```python
from build123d import *

# Parameters (mm, degrees)
F0_W     = 25.4
F0_H     = 25.4
F1_DEPTH = 25.4
F3_DEPTH = 23.368
F2_W     = 2.54
F2_H     = 15.24
F4_DEPTH = 20.32


with BuildPart() as f1:
    # F0 (on Top) → F1 (new body)
    with BuildSketch(Plane.XY):
        Rectangle(F0_W, F0_H)
    extrude(amount=F1_DEPTH)

    # F2 (on face) → F3 (cut)
    with BuildSketch(Plane(origin=(0, 0, 0), x_dir=(1, 0, 0), z_dir=(0, 0, -1))):
        Polygon((10.16, -7.62), (10.16, 7.62), (10.16, 10.668), (7.62, 10.668), (7.62, -10.668), (10.16, -10.668), align=None)
    extrude(amount=-F3_DEPTH, mode=Mode.SUBTRACT)

    # F2 (on face) → F4 (cut)
    with BuildSketch(Plane(origin=(0, 0, 0), x_dir=(1, 0, 0), z_dir=(0, 0, -1))):
        with Locations((11.43, 0)):
            Rectangle(F2_W, F2_H)
    extrude(amount=-F4_DEPTH, mode=Mode.SUBTRACT)


solid = f1.part
```
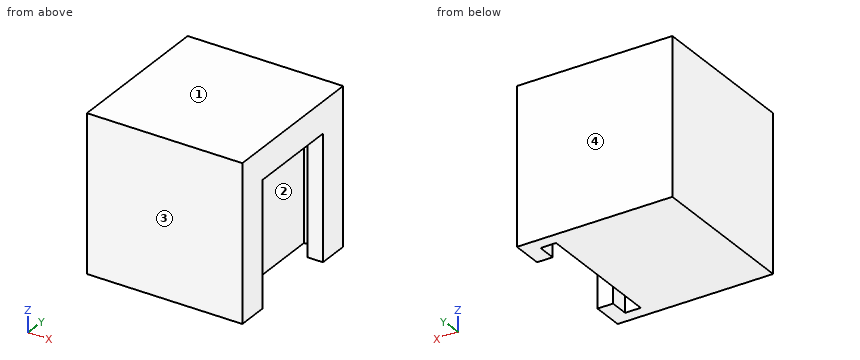
Check sheet for the modelled part. Datum: model origin and axes. Units: mm. Face numbers are marked on the shaded views. Coordinates: 2 decimals unless noted, no trailing zeros. Write each loop counter-clockwise with the first axis right and the second up, starting at its lowest first coordinate (ties: lowest second). Pieces come first, ordered by that corner, then holes. Notation, with made-up numbers: (11, 69.25) -> (55, 69.25) arc R32 ccw to (55, 97.25) -> close; hole circle Ø9 at (37, -3). An arc over 180 degrees is marked (long way). Use a Markdown table: item, result.
1. Sectioned sample at C-C (y = 9.5). Enter the section's corners in (x, z), plus the area to 3 significant figures.
Reported:
| item | result |
|---|---|
| outline | (-12.7, 0) -> (7.62, 0) -> (7.62, 23.37) -> (10.16, 23.37) -> (10.16, 0) -> (12.7, 0) -> (12.7, 25.4) -> (-12.7, 25.4) -> close |
| area | 586 mm2 |
2. Sectioned sample at A-A (z = 20.75). Enter the section's corners in (x, y).
Reported:
| item | result |
|---|---|
| outline | (-12.7, -12.7) -> (12.7, -12.7) -> (12.7, 12.7) -> (-12.7, 12.7) -> close; hole (7.62, -10.67) -> (10.16, -10.67) -> (10.16, 10.67) -> (7.62, 10.67) -> close |
3. Scan lines: line 1 along X through (y, z) = (-8.75, 21.75); line 2 along Y through (x, z) = (9.5, 16.5); line 3 along X through (y, z) = (-7.25, 1.75). Record each from-to range of solid material in increasing order.
Reported:
| item | result |
|---|---|
| line 1 | x = -12.7 to 7.62, 10.16 to 12.7 |
| line 2 | y = -12.7 to -10.67, 10.67 to 12.7 |
| line 3 | x = -12.7 to 7.62 |
4. Sectioned sample at B-B (x = 9.25). Enter the section's corners in (y, z).
Reported:
| item | result |
|---|---|
| outline | (-12.7, 0) -> (-10.67, 0) -> (-10.67, 23.37) -> (10.67, 23.37) -> (10.67, 0) -> (12.7, 0) -> (12.7, 25.4) -> (-12.7, 25.4) -> close |
5. Release check for a two-part mould opening along Y. For the marked faces 1, 2, 3 and 4 record: pulls with the +Y half, pulls with the -Y half, needs draft (parallel to the pull), parting line crosses it, or undercut.
Reported:
| item | result |
|---|---|
| face 1 | needs draft |
| face 2 | undercut |
| face 3 | pulls with the -Y half |
| face 4 | pulls with the +Y half |
6. Go/stop test with flat-tipped pins: pin 1 Ø1.5 at (y, z) = (-6, 7.5) entering from +X; pin 2 Ø3 at (x, y) = (11.5, 1) entering from -Z. Record where each tip stops, or that it passes through.
Reported:
| item | result |
|---|---|
| pin 1 | stops at x = 7.62 |
| pin 2 | stops at z = 20.32 |
